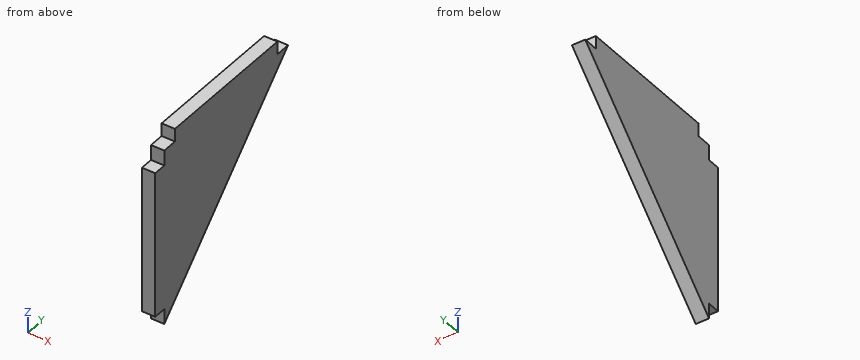
Autodesk Inventor part; units mm, degrees
ref_plane "YZ Plane" through (0, 0, 0) normal (1, 0, 0) x (0, 1, 0)
ref_plane "XZ Plane" through (0, 0, 0) normal (0, 1, 0) x (-1, 0, 0)
ref_plane "XY Plane" through (0, 0, 0) normal (0, 0, 1) x (1, 0, 0)
sketch "스케치1" plane through (0, 0, 0) normal (1, 0, 0) x (0, 1, 0)
  line L0 (0, -46.5) -> (46.5, 0)
  line L1 (0, -4) -> (-3.4, -4)
  line L2 (-3.4, -4) -> (-3.4, -42.5)
  line L3 (-3.4, -42.5) -> (0, -42.5)
  line L4 (0, 0) -> (0, -4)
  line L5 (0, -42.5) -> (0, -46.5)
  line L6 (42.5, 0) -> (42.5, 3.4)
  line L7 (42.5, 3.4) -> (4, 3.4)
  line L8 (4, 3.4) -> (4, 0)
  line L9 (46.5, 0) -> (42.5, 0)
  line L10 (4, 0) -> (0, 0)
  point P0 (4, 1.7)
  point P1 (0, -44.5)
  dimension "d1" = 46.5
  dimension "d2" = 38.5
  dimension "d4" = 38.5
  dimension "d5" = 3.4
  dimension "d6" = 4
  dimension "d7" = 3.4
  dimension "d8" = 46.5
extrude "돌출1" add sketch "스케치1" along normal blind 3.5
properties part number "supporter"
Could you check a few things on this model? Use its own coordinates, in mm. Give positions to 0.01 mm unless a question says otherwise; leave off trailing zeros. Loops run counter-clockwise (first coordinate to the right, second up) from the corner with the lowest first, then second, coordinate; pieces in that order, holes last. Notation, with made-up numbers: (-39, 20) - (6, 20) arc R31 cw to (6, 45) - close; hole circle Ø5 at (45, 49.25). An arc over 180 degrees is marked (long way). Answer in a Markdown table with one row per item. Add a question column.
Q1. If we section it at A-A (x = 0.7): List the corners of the cut face in (y, z) for me, plus the area to 3 significant figures.
Q2. Please list where these lines run through material, in increasing order: L1, parallel to Y at x = 0.9, z = -43; L2, parallel to Z at x = 0.8, y = 32; L3, parallel to Z at x = 2.75, y = 22. Write a range as from..to.
Q3. For pin 1 (1.5 mm diameter, centred on x = 3, y = 8.5, fed in from -Z); pin 2 (1.8 mm diameter, centred on x = 1.5, z = -45, fed in from -Y), each with a flat end and sliding along its axis, tell me the tip position at first contact or that it passes through.
Q4. If we section it at C-C (y = 37): List the corners of the cut face in (x, z) for me, plus the area to 4 significant figures.
Q5. If we section it at B-B (z = -31.5): List the corners of the cut face in (x, y) for me.
The answers:
| question | item | result |
|---|---|---|
| 1 | outline | (-3.4, -42.5) - (0, -42.5) - (0, -46.5) - (46.5, 0) - (42.5, 0) - (42.5, 3.4) - (4, 3.4) - (4, 0) - (0, 0) - (0, -4) - (-3.4, -4) - close |
| 1 | area | 1,340 mm^2 |
| 2 | L1 | y = 0..3.5 |
| 2 | L2 | z = -14.5..3.4 |
| 2 | L3 | z = -24.5..3.4 |
| 3 | pin 1 | stops at z = -38.75 |
| 3 | pin 2 | stops at y = 0 |
| 4 | outline | (0, -9.5) - (3.5, -9.5) - (3.5, 3.4) - (0, 3.4) - close |
| 4 | area | 45.15 mm^2 |
| 5 | outline | (0, -3.4) - (3.5, -3.4) - (3.5, 15) - (0, 15) - close |
